from build123d import *

# Parameters (mm, degrees)
SKETCH1_R           = 1.5
SKETCH1_R_2         = 15
BOSS_EXTRUDE1_DEPTH = 1
SKETCH2_R           = 25
BOSS_EXTRUDE2_DEPTH = 0.1
SKETCH3_R           = 15
CUT_EXTRUDE1_DEPTH  = 1


with BuildPart() as part:
    # Sketch1 → Boss-Extrude1 (new body)
    with BuildSketch(Plane.XY):
        with BuildLine():
            Line((-32.5, 40), (-32.5, -40))
            Line((-32.5, -40), (32.5, -40))
            Line((32.5, -40), (32.5, 40))
            ThreePointArc((32.5, 40), (0, 72.5), (-32.5, 40))
        make_face()
        with Locations((-30, -30)):
            Circle(SKETCH1_R, mode=Mode.SUBTRACT)
        with Locations((-30, 30)):
            Circle(SKETCH1_R, mode=Mode.SUBTRACT)
        with Locations((30, -30)):
            Circle(SKETCH1_R, mode=Mode.SUBTRACT)
        with Locations((30, 30)):
            Circle(SKETCH1_R, mode=Mode.SUBTRACT)
        with Locations((0, 30)):
            Circle(SKETCH1_R_2, mode=Mode.SUBTRACT)
    extrude(amount=BOSS_EXTRUDE1_DEPTH)

    # Sketch2 → Boss-Extrude2 (add)
    with BuildSketch(Plane.XY.offset(1)):
        with Locations((0, 30)):
            Circle(SKETCH2_R)
    extrude(amount=BOSS_EXTRUDE2_DEPTH)

    # Sketch3 → Cut-Extrude1 (cut)
    with BuildSketch(Plane(origin=(0, 0, 1), x_dir=(-1, 0, 0), z_dir=(0, 0, -1))):
        with Locations(Location((0, 30, 0), (0, 0, 180))):
            Circle(SKETCH3_R)
    extrude(amount=-CUT_EXTRUDE1_DEPTH, mode=Mode.SUBTRACT)


solid = part.part
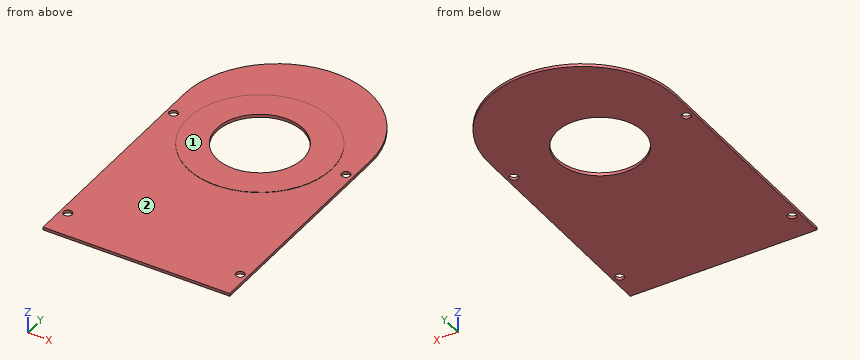
Work out the finished part from the listing and answer in its coordinate system (mm). Face numbers are marked on the shaded views. A direction names the side the tool comes from. Give positions to 0.01 mm unless a question says otherwise; leave off trailing zeros. Loops run counter-clockwise (first coordinate to the right, second up) from the corner with the lowest first, then second, coordinate; pieces in that order, holes last. Notation, with made-up numbers: (-7, 85.5) -> (14, 85.5) arc R24 ccw to (14, 114.5) -> close; hole circle Ø10 at (58.5, -17.75). An arc over 180 degrees is marked (long way). Use a Markdown table: item, result. Add a question column.
1) Each of these flat-tipped pins is pushed along its axis until it touches: P1, Ø2.5, axis at x = -30, y = 30, coming from the +Z side; P2, Ø3.5, axis at x = 30, y = 30, coming from the +Z side. Where does it stop, or does it pass through?
2) The part is cut by section B-B, the plane x = 0. Determine the outline of the cut face in (y, z).
3) The part is cut by section D-D, the plane x = 30. Determine the outline of the cut face in (y, z).
4) The part is cut by section A-A, the plane y = -30. Determine the outline of the cut face in (x, z), plus the area to 3 significant figures.
5) Which of the six approach directions +Z, -Z, +X, -X, +Y, -Y give full straight-line access (tool end or side, diameter ignored) to the marked faces 1 and 2?
6) The part is cut by section C-C, the plane y = 34. Determine the outline of the cut face in (x, z), plus the area to 3 significant figures.
7) Consider line 1 along Y through (x, z) = (0, 0.45); line 2 along X through (y, z) = (31, 0.4); line 3 along Z through (x, y) = (24.5, 9). Determine where each line is inside the solid, lowest interval first.
Reported:
| question | item | result |
|---|---|---|
| 1 | P1 | passes through |
| 1 | P2 | stops at z = 1 |
| 2 | outline | (-40, 0) -> (15, 0) -> (15, 1.1) -> (5, 1.1) -> (5, 1) -> (-40, 1) -> close; (45, 0) -> (72.5, 0) -> (72.5, 1) -> (55, 1) -> (55, 1.1) -> (45, 1.1) -> close |
| 3 | outline | (-40, 0) -> (-31.5, 0) -> (-31.5, 1) -> (-40, 1) -> close; (-28.5, 0) -> (28.5, 0) -> (28.5, 1) -> (-28.5, 1) -> close; (31.5, 0) -> (52.5, 0) -> (52.5, 1) -> (31.5, 1) -> close |
| 4 | outline | (-32.5, 0) -> (-31.5, 0) -> (-31.5, 1) -> (-32.5, 1) -> close; (-28.5, 0) -> (28.5, 0) -> (28.5, 1) -> (-28.5, 1) -> close; (31.5, 0) -> (32.5, 0) -> (32.5, 1) -> (31.5, 1) -> close |
| 4 | area | 59.0 mm^2 |
| 5 | face 1 | +Z, +X, -X, +Y, -Y |
| 5 | face 2 | +Z |
| 6 | outline | (-32.5, 0) -> (-14.46, 0) -> (-14.46, 1.1) -> (-24.68, 1.1) -> (-24.68, 1) -> (-32.5, 1) -> close; (14.46, 0) -> (32.5, 0) -> (32.5, 1) -> (24.68, 1) -> (24.68, 1.1) -> (14.46, 1.1) -> close |
| 6 | area | 38.1 mm^2 |
| 7 | line 1 | y = -40 to 15, 45 to 72.5 |
| 7 | line 2 | x = -32.5 to -31.12, -28.88 to -14.97, 14.97 to 28.88, 31.12 to 32.5 |
| 7 | line 3 | z = 0 to 1 |
